from build123d import *

# Parameters (mm, degrees)
F1_DEPTH = 10.16
F2_DEPTH = 4.2926
F3_R     = 5.08


with BuildPart() as f1:
    # F0 (on Front) → F1 (new body)
    with BuildSketch(Plane.XZ):
        with BuildLine():
            ThreePointArc((-1.3040083906, -12.6328762409), (-9.4021103543, -8.5375828479), (-12.6997273966, -0.0832108883))
            Line((-12.6997273966, -0.0832108883), (-25.3994547932, -0.1664217767))
            Line((-25.3994547932, -0.1664217767), (-25.3994547932, -12.6328762409))
            Line((-25.3994547932, -12.6328762409), (-1.3040083906, -12.6328762409))
        make_face()
        with BuildLine():
            Line((-25.3994547932, -0.1664217767), (-12.6997273966, -0.0832108883))
            ThreePointArc((-12.6997273966, -0.0832108883), (-10.061608872, 7.7494533295), (-3.162150516, 12.3000326875))
            Line((-3.162150516, 12.3000326875), (-25.3994547932, 12.3000326875))
            Line((-25.3994547932, 12.3000326875), (-25.3994547932, -0.1664217767))
        make_face()
        with BuildLine():
            Line((25.4005452068, 12.3000326875), (3.162150516, 12.3000326875))
            ThreePointArc((3.162150516, 12.3000326875), (10.0361673848, 7.7823739452), (12.7, 0))
            ThreePointArc((12.7, 0), (9.4300293361, -8.5067353738), (1.3040083906, -12.6328762409))
            Line((1.3040083906, -12.6328762409), (25.4005452068, -12.6328762409))
            Line((25.4005452068, -12.6328762409), (25.4005452068, 12.3000326875))
        make_face()
        with BuildLine():
            ThreePointArc((-3.162150516, 12.3000326875), (-10.061608872, 7.7494533295), (-12.6997273966, -0.0832108883))
            ThreePointArc((-12.6997273966, -0.0832108883), (-9.4021103543, -8.5375828479), (-1.3040083906, -12.6328762409))
            Line((-1.3040083906, -12.6328762409), (1.3040083906, -12.6328762409))
            ThreePointArc((1.3040083906, -12.6328762409), (9.4300293361, -8.5067353738), (12.7, 0))
            ThreePointArc((12.7, 0), (10.0361673848, 7.7823739452), (3.162150516, 12.3000326875))
            Line((3.162150516, 12.3000326875), (-3.162150516, 12.3000326875))
        make_face()
        Polygon((-2.7865785047, 5.9819127574), (3.7871991587, 5.4042041534), (6.5737776635, -0.5777086039), (2.7865785047, -5.9819127574), (-3.7871991587, -5.4042041534), (-6.2854766309, -0.0411835686), (-6.5737776635, 0.5777086039), align=None, mode=Mode.SUBTRACT)
        Polygon((6.5737776635, -0.5777086039), (3.7871991587, 5.4042041534), (-2.7865785047, 5.9819127574), (-6.5737776635, 0.5777086039), (-6.2854766309, -0.0411835686), (-3.7871991587, -5.4042041534), (2.7865785047, -5.9819127574), align=None)
        with BuildLine():
            Line((1.3040083906, -12.6328762409), (-1.3040083906, -12.6328762409))
            ThreePointArc((-1.3040083906, -12.6328762409), (0, -12.7), (1.3040083906, -12.6328762409))
        make_face()
        with BuildLine():
            ThreePointArc((3.162150516, 12.3000326875), (0, 12.7), (-3.162150516, 12.3000326875))
            Line((-3.162150516, 12.3000326875), (3.162150516, 12.3000326875))
        make_face()
    extrude(amount=F1_DEPTH)

    # F0 (on Front) → F2 (cut)
    with BuildSketch(Plane.XZ):
        Polygon((6.5737776635, -0.5777086039), (3.7871991587, 5.4042041534), (-2.7865785047, 5.9819127574), (-6.5737776635, 0.5777086039), (-6.2854766309, -0.0411835686), (-3.7871991587, -5.4042041534), (2.7865785047, -5.9819127574), align=None)
    extrude(amount=F2_DEPTH, mode=Mode.SUBTRACT)

    # F3
    f3_edges = [f1.edges().sort_by_distance(p)[0] for p in [
        (-25.399455, -5.08, 12.300033),
        (25.400545, -5.08, 12.300033),
        (25.400545, -5.08, -12.632876),
        (13.352277, -10.16, -12.632876),
        (-13.351732, -10.16, -12.632876),
        (0, -10.16, -12.7),
        (25.400545, -10.16, -0.166422),
        (14.281348, -10.16, 12.300033),
        (0, -10.16, 12.7),
        (-14.280803, -10.16, 12.300033),
        (-25.399455, -10.16, -0.166422),
        (-25.399455, -5.08, -12.632876),
    ]]
    fillet(f3_edges, radius=F3_R)


solid = f1.part
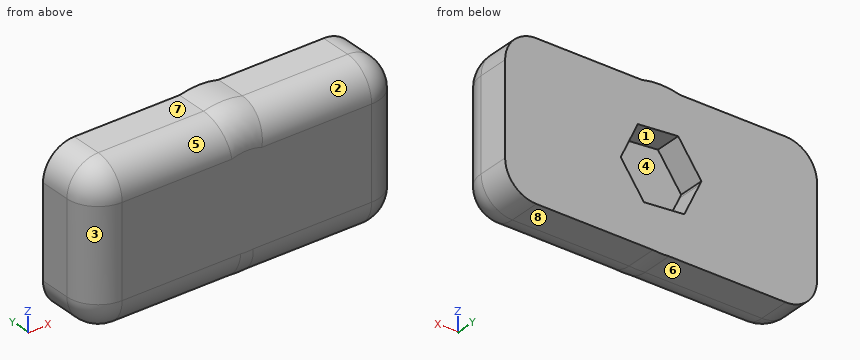
Here's how the part is built. I have some questions about the finished solid (model axes, mm). Face numbers are marked on the shaded views. A direction names the side the tool comes from. Round coordinates to 2 decimals unless told otherwise and drop trailing zeros. Order: outer loops, then holes, each group sorted by start corner. A loop starts at its lowest first (then second) coordinate and runs counter-clockwise, first axis right, second up. Notation, with made-up numbers: M 84,19.25 L 136,19.25 A28 ccw 136,40.25 Z; hole C -15,-27 d9. An arc over 180 degrees is marked long. One line per question, with ' | ' between items.
1) Imagine slicing it at D-D, the plane y = -6. Write out the boundary of the cut face in (x, z).
Checked values:
outline: M -25.32,-7.55 A5 ccw -20.32,-12.55 L -1.3,-12.55 A12.62 ccw 1.3,-12.55 L 20.32,-12.55 A5 ccw 25.32,-7.55 L 25.32,7.22 A5 ccw 20.32,12.22 L 3.15,12.22 A12.62 ccw -3.15,12.22 L -20.32,12.22 A5 ccw -25.32,7.22 Z
2) Imagine slicing it at B-B, the plane z = -4.75. Write out the boundary of the cut face in (x, y).
Checked values:
outline: M -25.4,-5.08 A5.08 ccw -20.32,-10.16 L 20.32,-10.16 A5.08 ccw 25.4,-5.08 L 25.4,0 L 3.65,0 L 3.65,-4.29 L -4.09,-4.29 L -4.09,0 L -25.4,0 Z
3) I'm going to push flat-ended pins straight in: pin 1 Ø5.5 at (x, y) = (-13.5, -3) entering from +Z; pin 2 Ø5.5 at (x, y) = (8, -3.5) entering from -Z; pin 3 Ø3.5 at (x, z) = (3, -2) entering from +Y; pin 4 Ø1 at (x, z) = (-9, 0) entering from +Y. Where does each tip first touch, or does it pass through?
Checked values:
pin 1: stops at z = 12.3 | pin 2: stops at z = -12.63 | pin 3: stops at y = -4.29 | pin 4: stops at y = 0
4) We'd pull the mould along X, two halves only. Please class the marked faces 1, 2 and 3: released by +X, released by -X, zero draft, split by the parting line, or undercut.
Checked values:
face 1: undercut | face 2: zero draft | face 3: released by -X
5) On a 3-axis mill with a long thin cutter (end or side, diameter ignored), from which of +Z, -Z, +X, -X, +Y, -Y can I reach the whole of each face in a straight line? I mean the marked faces 4, 5, 6, 7 and 8. Say none if no direction works.
Checked values:
face 4: +Y | face 5: +Z, -X, -Y | face 6: -Z, -X, +Y, -Y | face 7: +Z, -X, +Y, -Y | face 8: -Z, +X, +Y, -Y
6) Imagine slicing it at C-C, the plane x = -15.5. Write out the boundary of the cut face in (y, z).
Checked values:
outline: M -10.16,-7.55 A5.08 ccw -5.08,-12.63 L 0,-12.63 L 0,12.3 L -5.08,12.3 A5.08 ccw -10.16,7.22 Z
7) I need wall thicknesses on line 1 (Z direction, x = -4.5, y = -4); line 2 (Z direction, x = 14, y = -3.75); line 3 (X direction, y = -2.75, z = 3.5). Which ranges of each line are inside material? Lowest first, please.
Checked values:
line 1: z = -12.63 to -3.87, 3.54 to 12.3 | line 2: z = -12.63 to 12.3 | line 3: x = -25.4 to -4.53, 4.67 to 25.4
8) Imagine slicing it at A-A, the plane y = -1.75. Write out the boundary of the cut face in (x, z).
Checked values:
outline: M -25.4,-7.55 A5.08 ccw -20.32,-12.63 L -1.3,-12.63 A12.7 ccw 1.3,-12.63 L 20.32,-12.63 A5.08 ccw 25.4,-7.55 L 25.4,7.22 A5.08 ccw 20.32,12.3 L 3.16,12.3 A12.7 ccw -3.16,12.3 L -20.32,12.3 A5.08 ccw -25.4,7.22 Z; hole M -6.57,0.58 L -3.79,-5.4 L 2.79,-5.98 L 6.57,-0.58 L 3.79,5.4 L -2.79,5.98 Z
